```python
from build123d import *

# Parameters (mm, degrees)
SKETCH_W     = 13
SKETCH_H     = 13
PAD_DEPTH    = 7
CHAMFER_SIZE = 2
POCKET_DEPTH = 7


with BuildPart() as part:
    # Sketch → Pad (new body)
    with BuildSketch(Plane.XY):
        with Locations((6.5, 6.5)):
            Rectangle(SKETCH_W, SKETCH_H)
    extrude(amount=PAD_DEPTH)

    # Chamfer
    chamfer_edges = [part.edges().sort_by_distance(p)[0] for p in [
        (0, 6.5, 7),
        (6.5, 13, 7),
        (6.5, 0, 7),
        (13, 6.5, 7),
    ]]
    chamfer(chamfer_edges, length=CHAMFER_SIZE)

    # Sketch002 (on Face4 of Chamfer) → Pocket (cut)
    with BuildSketch(Plane(origin=(0, 0, 0), x_dir=(1, 0, 0), z_dir=(0, 0, -1))):
        with BuildLine():
            Line((0, 0), (0, -0.5))
            ThreePointArc((0.5, 0), (0.146447, -0.146447), (0, -0.5))
            Line((0, 0), (0.5, 0))
        make_face()
        with BuildLine():
            Line((13, 0), (12.5, 0))
            ThreePointArc((13, -0.5), (12.853553, -0.146447), (12.5, 0))
            Line((13, 0), (13, -0.5))
        make_face()
        with BuildLine():
            Line((0, -12.5), (0, -13))
            Line((0, -13), (0.5, -13))
            ThreePointArc((0, -12.5), (0.146447, -12.853553), (0.5, -13))
        make_face()
        with BuildLine():
            Line((13, -12.5), (13, -13))
            Line((13, -13), (12.5, -13))
            ThreePointArc((12.5, -13), (12.853553, -12.853553), (13, -12.5))
        make_face()
    extrude(amount=-POCKET_DEPTH, mode=Mode.SUBTRACT)


solid = part.part
```
Could you check a few things on this model? Use its own coordinates, in mm. Round coordinates to 2 decimals unless told otherwise and drop trailing zeros. Loops run counter-clockwise (first coordinate to the right, second up) from the corner with the lowest first, then second, coordinate; pieces in that order, holes last.
Q1. I want a section at C-C (z = 5.5). Write out the boundary of the cut face in (x, y), and give its area (3 significant figures).
Q2. For P1, Ø1, axis at x = 3.5, y = 1.5, coming from the -Z side, with a flat end and sliding along its axis, tell me the tip position at first contact or that it passes through.
Q3. Please list where these lines run through material, in increasing order: L1, parallel to X at y = 11, z = 5.5; L2, parallel to Z at x = 1.75, y = 2.75; L3, parallel to Z at x = 4.75, y = 12.25.
Q4. I want a section at A-A (x = 1.75). Write out the boundary of the cut face in (y, z).
Q5. I want a section at B-B (y = 11.75). Write out the boundary of the cut face in (x, z).
Answer below:
1. outline: (0.5, 0.5) - (12.5, 0.5) - (12.5, 12.5) - (0.5, 12.5) - close
1. area: 144 mm2
2. P1: stops at z = 0
3. L1: x = 0.5 to 12.5
3. L2: z = 0 to 6.75
3. L3: z = 0 to 5.75
4. outline: (0, 0) - (13, 0) - (13, 5) - (11.25, 6.75) - (1.75, 6.75) - (0, 5) - close
5. outline: (0, 0) - (13, 0) - (13, 5) - (11.75, 6.25) - (1.25, 6.25) - (0, 5) - close
